```python
from build123d import *

# Parameters (mm, degrees)
EXTRUDE_1_DEPTH     = 15
SKETCH_2_R          = 3.5
CUT_EXTRUDE_2_DEPTH = 15
EXTRUDE_START       = -15
EXTRUDE_2_DEPTH     = 15
CUT_EXTRUDE_3_REACH = 164.969
SKETCH_4_R          = 3
EXTRUDE_3_DEPTH     = 15
FILLET_2_R          = 100
FILLET_3_R          = 100
SKETCH_6_R          = 3
CUT_EXTRUDE_4_DEPTH = 30
CUT_EXTRUDE_5_DEPTH = 4.5


with BuildPart() as part:
    # 草图1 → 凸台-拉伸1 (new body)
    with BuildSketch(Plane.XY):
        with BuildLine():
            Line((-90.35, 0), (-110, 0))
            ThreePointArc((-110, 0), (0, 110), (110, 0))
            Line((110, 0), (90.35, 0))
            ThreePointArc((90.35, 0), (0, 90.35), (-90.35, 0))
        make_face()
    extrude(amount=EXTRUDE_1_DEPTH)

    # 草图2 → 切除-拉伸2 (cut)
    with BuildSketch(Plane.XY.offset(15)):
        with Locations((38.268343237, 92.387953251)):
            Circle(SKETCH_2_R)
        with Locations((92.387953251, 38.268343237)):
            Circle(SKETCH_2_R)
        with Locations((92.387953251, -38.268343237)):
            Circle(SKETCH_2_R)
        with Locations((38.268343237, -92.387953251)):
            Circle(SKETCH_2_R)
        with Locations((-38.268343237, -92.387953251)):
            Circle(SKETCH_2_R)
        with Locations((-92.387953251, -38.268343237)):
            Circle(SKETCH_2_R)
        with Locations((-92.387953251, 38.268343237)):
            Circle(SKETCH_2_R)
        with Locations((-38.268343237, 92.387953251)):
            Circle(SKETCH_2_R)
    extrude(amount=-CUT_EXTRUDE_2_DEPTH, mode=Mode.SUBTRACT)

    # 草图3 → 凸台-拉伸2 (add)
    with BuildSketch(Plane.XY.offset(15).offset(EXTRUDE_START)):
        with BuildLine():
            Line((-110, 0), (-129.343495463, 0))
            Line((-129.343495463, 0), (-129.343495463, 12))
            Line((-129.343495463, 12), (-109.343495463, 12))
            ThreePointArc((-109.343495463, 12), (-109.83575124, 6.008972421), (-110, 0))
        make_face()
        with BuildLine():
            Line((129.343495463, 12), (109.343495463, 12))
            ThreePointArc((109.343495463, 12), (109.83575124, 6.008972421), (110, 0))
            Line((110, 0), (129.343495463, 0))
            Line((129.343495463, 0), (129.343495463, 12))
        make_face()
    extrude(amount=EXTRUDE_2_DEPTH)

    # 草图4 → 切除-拉伸3 (cut, up to next)
    with BuildSketch(Plane(origin=(0, 12, 0), x_dir=(1, 0, 0), z_dir=(0, 1, 0)), mode=Mode.PRIVATE) as cut_extrude_3_sk1:
        with Locations(Location((-119.343495463, -7.5, 0), (0, 0, 270))):
            Circle(SKETCH_4_R)
    cut_extrude_3_tool1 = extrude(cut_extrude_3_sk1.sketch, amount=-CUT_EXTRUDE_3_REACH, mode=Mode.PRIVATE) & part.part
    cut_extrude_3 = cut_extrude_3_tool1.solids().sort_by_distance((-119.343495, 12, 7.5))[0]
    add(cut_extrude_3, mode=Mode.SUBTRACT)

    # 镜向1: 切除-拉伸3 across plane
    add(cut_extrude_3.mirror(Plane.ZY), mode=Mode.SUBTRACT)

    # 草图5 → 凸台-拉伸3 (add)
    with BuildSketch(Plane.XY.offset(15).offset(EXTRUDE_START)):
        with BuildLine():
            Line((-90, 130), (90, 130))
            Line((90, 130), (90, 110))
            Line((90, 110), (107.821782178, 21.782178218))
            ThreePointArc((107.821782178, 21.782178218), (0, 110), (-107.821782178, 21.782178218))
            Line((-107.821782178, 21.782178218), (-90, 110))
            Line((-90, 110), (-90, 130))
        make_face()
    extrude(amount=EXTRUDE_3_DEPTH)

    # 圆角2
    fillet_2_edges = [part.edges().sort_by_distance(p)[0] for p in [
        (90, 110, 7.5),
    ]]
    fillet(fillet_2_edges, radius=FILLET_2_R)

    # 圆角3
    fillet_3_edges = [part.edges().sort_by_distance(p)[0] for p in [
        (-90, 110, 7.5),
    ]]
    fillet(fillet_3_edges, radius=FILLET_3_R)

    # 草图6 → 切除-拉伸4 (cut)
    with BuildSketch(Plane(origin=(0, 130, 0), x_dir=(1, 0, 0), z_dir=(0, 1, 0))):
        with Locations(Location((-70, -7.5, 0), (0, 0, 270))):
            Circle(SKETCH_6_R)
    cut_extrude_4 = extrude(amount=-CUT_EXTRUDE_4_DEPTH, mode=Mode.SUBTRACT)

    # 草图7 → 切除-拉伸5 (cut)
    with BuildSketch(Plane(origin=(0, 110, 0), x_dir=(1, 0, 0), z_dir=(0, 1, 0))):
        Polygon((-74.25, -9.953738644), (-74.25, -15), (-65.75, -15), (-65.75, -9.953738644), (-65.75, -5.046261356), (-70, -2.592522712), (-74.25, -5.046261356), align=None)
    cut_extrude_5 = extrude(amount=CUT_EXTRUDE_5_DEPTH, mode=Mode.SUBTRACT)

    # 镜向2: 切除-拉伸4, 切除-拉伸5 across plane
    add(cut_extrude_4.mirror(Plane.ZY), mode=Mode.SUBTRACT)
    add(cut_extrude_5.mirror(Plane.ZY), mode=Mode.SUBTRACT)


solid = part.part
```
Work out the finished part from the listing and answer in its coordinate system (mm). A direction names the side the tool comes from. Coordinates: 2 decimals unless noted, no trailing zeros. Loops run counter-clockwise (first coordinate to the right, second up) from the corner with the lowest first, then second, coordinate; pieces in that order, holes last. Notation, with made-up numbers: (66.25, 89.5) - (95.25, 89.5) arc R9 ccw to (95.25, 95.5) - close; hole circle Ø5 at (59.5, 82.5). An arc over 180 degrees is marked (long way). Use a Markdown table: item, result.
Item 1: Find section D-D, the plane x = -80. Determine the outline of the cut face in (y, z).
Evaluation:
| item | result |
|---|---|
| outline | (41.99, 0) - (130, 0) - (130, 15) - (41.99, 15) - close |
Item 2: Consider probe 1 along X at (y, z) = (103.25, 7.5); probe 2 along X at (y, z) = (93.5, 6.5); probe 3 along X at (y, z) = (9, 5.75). Determine where each line is inside the solid, lowest interval first. Write a range as from..to.
Evaluation:
| item | result |
|---|---|
| probe 1 | x = -91.41..-73, -67..67, 73..91.41 |
| probe 2 | x = -93.33..-41.59, -34.95..34.95, 41.59..93.33 |
| probe 3 | x = -129.34..-121.78, -116.91..-89.9, 89.9..116.91, 121.78..129.34 |
Item 3: Find section C-C, the plane x = 0. Determine the outline of the cut face in (y, z), and give its area (3 significant figures).
Evaluation:
| item | result |
|---|---|
| outline | (90.35, 0) - (130, 0) - (130, 15) - (90.35, 15) - close |
| area | 595 mm2 |
Item 4: The mould has two halves that part along Z. Classify faces 6 (the flat face through (2, 95, 15)), 7 (the flat face through (65.75, 112, 10)), 8 (the cylindrical face through (72.662, 122.358, 8.884)): +Z half, -Z half, draft (parallel to the pull), parting line (faces both ways), or undercut.
Evaluation:
| item | result |
|---|---|
| face 6 | +Z half |
| face 7 | draft |
| face 8 | undercut |
Item 5: Find section A-A, the plane y = 60. Determine the outline of the cut face in (x, z).
Evaluation:
| item | result |
|---|---|
| outline | (-100.1, 0) - (-67.55, 0) - (-67.55, 15) - (-100.1, 15) - close; (67.55, 0) - (100.1, 0) - (100.1, 15) - (67.55, 15) - close |
Item 6: Given pin 1 Ø8 at (x, z) = (57, 7.5) entering from -Y; pin 2 Ø1.8 at (x, z) = (-71, 9) entering from +Y; pin 3 Ø4 at (y, z) = (55.5, 6) entering from -X, each flat-ended and moving along its own axis, determine where each tip first touches the part or whether it passes through.
Evaluation:
| item | result |
|---|---|
| pin 1 | stops at y = 66.65 |
| pin 2 | stops at y = 100 |
| pin 3 | stops at x = -101.41 |
Item 7: Find section B-B, the plane z = 7.5. State how many separate pieces and enclosed holes the cut face has, and give its area (3 significant figures).
Evaluation:
| item | result |
|---|---|
| separate pieces | 3 |
| enclosed holes | 4 |
| area | 12,800 mm2 |
Item 8: For faces 1 (the flat face through (74.25, 112, 10)), 2 (the flat face through (-70, 100, 7)), 3 (the flat face through (90, 125, 7)), 4 (the flat face through (-110, 0, 7)), 5 (the flat face through (-119, 12, 4)), determine the directions among +Z, -Z, +X, -X, +Y, -Y from which every point of the face is accessible in a straight line to the end or side of a thin tool.
Evaluation:
| item | result |
|---|---|
| face 1 | +Z |
| face 2 | +Y |
| face 3 | +Z, -Z, +X, +Y |
| face 4 | +Z, -Z, +X, -X, -Y |
| face 5 | +Z, -Z, -X, +Y |
